Input: part model. Units: mm. Frame: model coordinates. Face numbers are marked on the shaded views. A direction names the side the tool comes from. Coordinates: 2 decimals unless noted, no trailing zeros. Loops run counter-clockwise (first coordinate to the right, second up) from the corner with the lowest first, then second, coordinate; pieces in that order, holes last. Notation, with made-up numbers: (-33.5, 48.5) - (2.5, 48.5) arc R23 cw to (2.5, 83.5) - close; hole circle Ø5 at (-36, 48). An arc over 180 degrees is marked (long way). Use a Markdown table: item, result. Add a question column.
1. Section query A-A on y = -5.5. Return the cut outline in (x, z).
2. Section query D-D on y = -9. Return the cut outline in (x, z), then the cut area to 3 significant figures.
3. Section query B-B on z = -6.75. Return the cut outline in (x, y), then the cut area to 3 significant figures.
4. Draft query along X for the marked faces 3 and 4. Return one class per face: released by +X, released by -X, zero draft, split by the parting line, or undercut.
5. Contact query for flat-ended pins moving along their axis: P1, Ø10, axis at x = -5.5, y = 8.5, coming from the -Z side; P2, Ø2.5, axis at x = 6, y = -5.5, coming from the +Z side. Output: stop coordinate, or through.
6. Ray query, L1, parallel to Y at x = -6, z = -0.5; L2, parallel to Y at x = 0, z = -7.5; L3, parallel to Z at x = 0, y = 10.5. Return the intervals inside material, ascending. Write a range as [from, to].
7. Section query C-C on x = -2.25. Return the cut outline in (y, z), then the cut area to 3 significant figures.
8. Access query for the marked faces 1 and 2. Directions: +Z, -Z, +X, -X, +Y, -Y. A direction counts if a zero-diameter tool reaches every point of the face in a straight line with its end or side. Return the directions, or none.
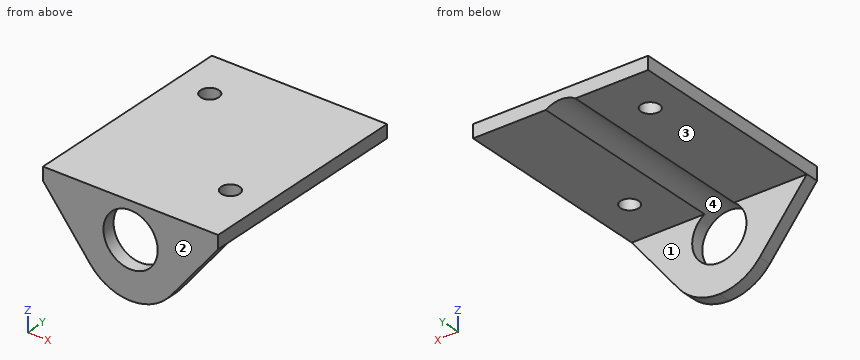
```python
from build123d import *

# Parameters (mm, degrees)
F0_W     = 20
F0_H     = 25
F0_R     = 1.05
F1_DEPTH = 1.5
F2_W     = 20
F2_H     = 1.5
F3_DEPTH = 9
F4_R     = 3.1
F5_DEPTH = 30


with BuildPart() as f1:
    # F0 (on Top) → F1 (new body)
    with BuildSketch(Plane.XY):
        Rectangle(F0_W, F0_H)
        with Locations((6, -5.5)):
            Circle(F0_R, mode=Mode.SUBTRACT)
        with Locations((-6, 7)):
            Circle(F0_R, mode=Mode.SUBTRACT)
    extrude(amount=-F1_DEPTH)

    # F2 (on face) → F3 (join)
    with BuildSketch(Plane(origin=(0, 0, -1.5), x_dir=(1, 0, 0), z_dir=(0, 0, -1))):
        with Locations((0, 11.75)):
            Rectangle(F2_W, F2_H)
    extrude(amount=F3_DEPTH)

    # F4 (on face) → F5 (cut)
    with BuildSketch(Plane.XZ.offset(12.5)):
        with Locations((0, -4.1)):
            Circle(F4_R)
        with BuildLine():
            Line((-4.618965, -8.270854), (-10, -1.5))
            Line((-10, -1.5), (-10, -10.5))
            Line((-10, -10.5), (0, -10.5))
            ThreePointArc((0, -10.5), (-2.564368, -9.913569), (-4.618965, -8.270854))
        make_face()
        with BuildLine():
            ThreePointArc((4.618965, -8.270854), (2.564368, -9.913569), (0, -10.5))
            Line((0, -10.5), (10, -10.5))
            Line((10, -10.5), (10, -1.5))
            Line((10, -1.5), (4.618965, -8.270854))
        make_face()
    extrude(amount=-F5_DEPTH, mode=Mode.SUBTRACT)


solid = f1.part
```
Resolved:
| question | item | result |
|---|---|---|
| 1 | outline | (-10, -1.5) - (-1.69, -1.5) arc R3.1 cw to (1.69, -1.5) - (4.95, -1.5) - (4.95, 0) - (-10, 0) - close; (7.05, -1.5) - (10, -1.5) - (10, 0) - (7.05, 0) - close |
| 2 | outline | (-10, -1.5) - (-1.69, -1.5) arc R3.1 cw to (1.69, -1.5) - (10, -1.5) - (10, 0) - (-10, 0) - close |
| 2 | area | 28.9 mm² |
| 3 | outline | (-5.83, -12.5) - (-1.61, -12.5) - (-1.61, -11) - (-5.83, -11) - close; (1.61, -12.5) - (5.83, -12.5) - (5.83, -11) - (1.61, -11) - close |
| 3 | area | 12.7 mm² |
| 4 | face 3 | zero draft |
| 4 | face 4 | undercut |
| 5 | P1 | z = -1.5 |
| 5 | P2 | z = 0 |
| 6 | L1 | [-12.5, 5.95], [8.05, 12.5] |
| 6 | L2 | [-12.5, -11] |
| 6 | L3 | [-1, 0] |
| 7 | outline | (-12.5, -10.05) - (-11, -10.05) - (-11, -6.23) - (-12.5, -6.23) - close; (-12.5, -1.97) - (-11, -1.97) - (-11, -1.5) - (12.5, -1.5) - (12.5, 0) - (-12.5, 0) - close |
| 7 | area | 43.9 mm² |
| 8 | face 1 | -Z, +X, -X, +Y |
| 8 | face 2 | +Z, -Z, +X, -X, -Y |
